Read the model definition and answer for the solid it produces. Units are mm, in the model's axes. A direction names the side the tool comes from. Give positions to 0.01 mm unless a question says otherwise; leave off trailing zeros. Order: outer loops, then holes, each group sorted by start corner. A loop starts at its lowest first (then second) coordinate and runs counter-clockwise, first axis right, second up.
```python
from build123d import *

# Parameters (mm, degrees)
F0_R     = 7.55
F1_DEPTH = 18.7
F2_R     = 10.9
F3_DEPTH = 2.3
F4_DEPTH = 0.2
F5_R     = 10.9
F6_DEPTH = 2.7
F7_R     = 5.15
F8_DEPTH = 50
F9_R     = 2


with BuildPart() as f1:
    # F0 (on Front) → F1 (new body)
    with BuildSketch(Plane.XZ):
        Circle(F0_R)
    extrude(amount=F1_DEPTH)

    # F2 (on face) → F3 (join)
    with BuildSketch(Plane(origin=(0, 0, 0), x_dir=(-1, 0, 0), z_dir=(0, 1, 0))):
        Circle(F2_R)
    extrude(amount=-F3_DEPTH)

    # F2 (on face) → F4 (join)
    with BuildSketch(Plane(origin=(0, 0, 0), x_dir=(-1, 0, 0), z_dir=(0, 1, 0))):
        Circle(F2_R)
    extrude(amount=F4_DEPTH)

    # F5 (on face) → F6 (join)
    with BuildSketch(Plane.XZ.offset(18.7)):
        Circle(F5_R)
    extrude(amount=-F6_DEPTH)

    # F7 (on Front) → F8 (cut, symmetric)
    with BuildSketch(Plane.XZ):
        Circle(F7_R)
    extrude(amount=F8_DEPTH, both=True, mode=Mode.SUBTRACT)

    # F9
    f9_edges = [f1.edges().sort_by_distance(p)[0] for p in [
        (-7.55, -2.3, 0),
        (-7.55, -16, 0),
    ]]
    fillet(f9_edges, radius=F9_R)


solid = f1.part
```
1) The part is cut by section A-A on x = 0. Determine the outline of the cut face in (y, z).
Final values:
outline: (-18.7, -10.9) - (-16, -10.9) - (-16, -9.55) arc R2 cw to (-14, -7.55) - (-4.3, -7.55) arc R2 cw to (-2.3, -9.55) - (-2.3, -10.9) - (0.2, -10.9) - (0.2, -5.15) - (-18.7, -5.15) - close; (-18.7, 5.15) - (0.2, 5.15) - (0.2, 10.9) - (-2.3, 10.9) - (-2.3, 9.55) arc R2 cw to (-4.3, 7.55) - (-14, 7.55) arc R2 cw to (-16, 9.55) - (-16, 10.9) - (-18.7, 10.9) - close
2) A tool of negligible diameter and unlimited length cuts with its end or side. For faces 4 (the face through (10.4, -17.37, 3.27)), 5 (the face through (0, -2.3, -10)), from which of +Z, -Z, +X, -X, +Y, -Y can it reach the whole face along a straight path? Write none if from no direction.
Final values:
face 4: +Y, -Y
face 5: none
3) The part is cut by section D-D on y = -3. Determine the outline of the cut face in (x, z), and give its area (3 significant figures).
Final values:
outline: circle Ø16.06 at (0, 0); hole circle Ø10.3 at (0, 0)
area: 119 mm2
4) Given pin 1 (4 mm diameter, centred on y = -4, z = 8.5, fed in from +X); pin 2 (1.5 mm diameter, centred on x = 2.5, y = -13.5, fed in from -Z); pin 3 (2 mm diameter, centred on y = -16, z = 3.5, fed in from +X), each flat-ended and moving along its own axis, determine where each tip first touches the part or whether it passes through.
Final values:
pin 1: stops at x = 7.96
pin 2: stops at z = -7.34
pin 3: stops at x = 10.61
5) The part is cut by section C-C on y = -12. Determine the outline of the cut face in (x, z).
Final values:
outline: circle Ø15.1 at (0, 0); hole circle Ø10.3 at (0, 0)
6) For a pull along Z with two mould halves and no side action, classify faces 1 (the face through (-1.64, -9.08, -7.37)), 2 (the face through (4.91, -9.38, 1.55)), 3 (the face through (2, -18.7, -5)) as released by +Z, released by -Z, zero draft, split by the parting line, or undercut.
Final values:
face 1: split by the parting line
face 2: undercut
face 3: zero draft
7) Consider L1, parallel to Z at x = 0, y = -6.5; L2, parallel to Y at x = -9, z = -6; L3, parallel to Y at x = 8, z = -4. Determine where each line is inside the solid, lowest interval first.
Final values:
L1: z = -7.55 to -5.15, 5.15 to 7.55
L2: y = -18.7 to -16, -2.3 to 0.2
L3: y = -18.7 to -15.91, -2.39 to 0.2
8) The part is cut by section B-B on z = 0. Determine the outline of the cut face in (x, y).
Final values:
outline: (-10.9, -18.7) - (-5.15, -18.7) - (-5.15, 0.2) - (-10.9, 0.2) - (-10.9, -2.3) - (-9.55, -2.3) arc R2 cw to (-7.55, -4.3) - (-7.55, -14) arc R2 cw to (-9.55, -16) - (-10.9, -16) - close; (5.15, -18.7) - (10.9, -18.7) - (10.9, -16) - (9.55, -16) arc R2 cw to (7.55, -14) - (7.55, -4.3) arc R2 cw to (9.55, -2.3) - (10.9, -2.3) - (10.9, 0.2) - (5.15, 0.2) - close
